```python
from build123d import *

# Parameters (mm, degrees)
SKETCH1_W                  = 210
SKETCH1_H                  = 40
BOSS_EXTRUDE1_DEPTH        = 3
F_3_0_3_DIAMETER_HOLE2_D   = 3
F_13_0_13_DIAMETER_HOLE1_D = 13


with BuildPart() as part:
    # Sketch1 → Boss-Extrude1 (new body)
    with BuildSketch(Plane.XY):
        with Locations((95, 0)):
            Rectangle(SKETCH1_W, SKETCH1_H)
    extrude(amount=BOSS_EXTRUDE1_DEPTH)

    # Ø3.0 (3) Diameter Hole2 (through all)
    with Locations(Plane(origin=(0, 0, 0), x_dir=(-1, 0, 0), z_dir=(0, 0, -1))):
        with Locations((-3, 8), (-11, 0), (5, 0), (-3, -8), (-3, 0)):
            Hole(F_3_0_3_DIAMETER_HOLE2_D / 2)

    # Ø13.0 (13) Diameter Hole1 (through all)
    with Locations(Plane.XY.offset(3)):
        with Locations((90, 0), (180, 0)):
            Hole(F_13_0_13_DIAMETER_HOLE1_D / 2)


solid = part.part
```
CAD build for the part. Positions are in the model's coordinates, mm. Give positions to 0.01 mm unless a question says otherwise; leave off trailing zeros. Write each loop counter-clockwise with the first axis right and the second up, starting at its lowest first coordinate (ties: lowest second). Pieces come first, ordered by that corner, then holes. Notation, with made-up numbers: M -19.5,-16.5 L 7.5,-16.5 A25 cw 7.5,20.5 Z; hole C 67,59 d5. An arc over 180 degrees is marked long. Return JSON: item names as keys, results as strings. Group by question number.
(1) Band-saw the part on A-A (z = 2.4). Give the cut face in (x, y).
(2) Flat gauge pin, fed straight in: pin 1 Ø8 at (x, y) = (180, 0) entering from +Z. Where does the tip first touch, or does it go through?
(3) Mould opens along X. For faces 1 (the face through (94, 9, 3)), 2 (the face through (186.494, 0.286, 1.479)) say: pulls with the +X half, pulls with the -X half, needs draft (parallel to the pull), parting line crosses it, or undercut.
(4) Drill centre lines: L1, parallel to Y at x = 180, z = 1.6; L2, parallel to X at y = 2.5, z = 0.8; L3, parallel to Y at x = 11, z = 1.6. Where is each one in solid material? Low to high. Write a range as [from, to].
Entries:
{
 "1": {"outline": "M -10,-20 L 200,-20 L 200,20 L -10,20 Z; hole C -5,0 d3; hole C 3,-8 d3; hole C 3,0 d3; hole C 3,8 d3; hole C 11,0 d3; hole C 90,0 d13; hole C 180,0 d13"},
 "2": {"pin 1": "passes through"},
 "3": {"face 1": "needs draft", "face 2": "undercut"},
 "4": {"L1": "y = [-20, -6.5], [6.5, 20]", "L2": "x = [-10, 84], [96, 174], [186, 200]", "L3": "y = [-20, -1.5], [1.5, 20]"}
}
